For this review, take the finished solid that the model builds, in its own axes (mm). Face numbers are marked on the shaded views. Give positions to 0.01 mm unless a question says otherwise; leave off trailing zeros. Loops run counter-clockwise (first coordinate to the right, second up) from the corner with the lowest first, then second, coordinate; pieces in that order, holes last. Notation, with made-up numbers: (31, 45) - (40, 45) arc R35 cw to (40, 82) - close; hole circle Ø8 at (2.5, -32.75). An arc over 180 degrees is marked (long way). Put each result on its own line as item: value. Start each with the question number.
from build123d import *

# Parameters (mm, degrees)
SKETCH1_W             = 9.525
SKETCH1_H             = 142.875
BOSS_EXTRUDE1_DEPTH   = 1.5875
BOSS_EXTRUDE1_2_DEPTH = 1.5875
SKETCH2_W             = 4.7625
SKETCH2_H             = 142.875
BOSS_EXTRUDE2_DEPTH   = 59.055
SKETCH3_W             = 127
SKETCH3_H             = 38.1
CUT_EXTRUDE1_DEPTH    = 164.834934713
SKETCH4_R             = 26.2255
SKETCH4_R_2           = 22.225
BOSS_EXTRUDE3_DEPTH   = 4.7625
FILLET1_R             = 6.35
FILLET4_R             = 6.35
SKETCH5_W             = 44.45
SKETCH5_H             = 1.5875
BOSS_EXTRUDE4_DEPTH   = 142.875


with BuildPart() as part:
    # Sketch1 → Boss-Extrude1 (new body)
    with BuildSketch(Plane(origin=(0, 0, 0), x_dir=(1, 0, 0), z_dir=(0, 1, 0))):
        with Locations((4.7625, 71.4375)):
            Rectangle(SKETCH1_W, SKETCH1_H)
    extrude(amount=BOSS_EXTRUDE1_DEPTH)



with BuildPart() as body_2:
    # Sketch1 → Boss-Extrude1 2 (new body)
    with BuildSketch(Plane(origin=(0, 0, 0), x_dir=(1, 0, 0), z_dir=(0, 1, 0))):
        with Locations((47.6885, 71.4375)):
            Rectangle(SKETCH1_W, SKETCH1_H)
    extrude(amount=BOSS_EXTRUDE1_2_DEPTH)


with BuildPart() as part_1:
    add(part.part)

    add(body_2.part)  # Boss-Extrude2 merges body 2
    # Sketch2 → Boss-Extrude2 (add)
    with BuildSketch(Plane(origin=(0, 1.5875, 0), x_dir=(1, 0, 0), z_dir=(0, 1, 0))):
        with Locations((2.38125, 71.4375)):
            Rectangle(SKETCH2_W, SKETCH2_H)
        with Locations((50.06975, 71.4375)):
            Rectangle(SKETCH2_W, SKETCH2_H)
    extrude(amount=BOSS_EXTRUDE2_DEPTH)

    # Sketch3 → Cut-Extrude1 (cut, through all)
    with BuildSketch(Plane.ZY):
        with Locations((-71.4375, 30.32125)):
            Rectangle(SKETCH3_W, SKETCH3_H)
    extrude(amount=-CUT_EXTRUDE1_DEPTH, mode=Mode.SUBTRACT)

    # Sketch4 → Boss-Extrude3 (add)
    with BuildSketch(Plane(origin=(0, 0, -142.875), x_dir=(-1, 0, 0), z_dir=(0, 0, -1))):
        with Locations((-26.2255, 30.32125)):
            Circle(SKETCH4_R)
        with Locations((-26.2255, 30.32125)):
            Circle(SKETCH4_R_2, mode=Mode.SUBTRACT)
    extrude(amount=-BOSS_EXTRUDE3_DEPTH)

    # Fillet1
    # the kernel refuses this fillet: 6.35 mm, written as the material it takes off along each edge
    with BuildSketch(Plane(origin=(52.451, 0, -158.75), x_dir=(0, 1, 0), z_dir=(0, 0, 1)), Plane(origin=(0, 0, -158.75), x_dir=(1, 0, 0), z_dir=(0, 0, 1))) as fillet1_piece_1:
        with BuildLine():
            CenterArc((FILLET1_R, FILLET1_R), FILLET1_R, 180, 90)
            Line((0, FILLET1_R), (-FILLET1_R * 0.02, FILLET1_R))
            Line((-FILLET1_R * 0.02, FILLET1_R), (-FILLET1_R * 0.02, -FILLET1_R * 0.02))
            Line((-FILLET1_R * 0.02, -FILLET1_R * 0.02), (FILLET1_R, -FILLET1_R * 0.02))
            Line((FILLET1_R, -FILLET1_R * 0.02), (FILLET1_R, 0))
        make_face()
    extrude(amount=174.625, mode=Mode.SUBTRACT)
    with BuildSketch(Plane(origin=(0, 60.6425, -158.245902655), x_dir=(1, 0, 0), z_dir=(0, 0, 1))) as fillet1_piece_2:
        with BuildLine():
            CenterArc((6.35, -6.148361062), FILLET1_R, 104.477512186, 75.522487814)
            Line((0, -6.148361062), (-0.127, -6.148361062))
            Line((-0.127, -6.148361062), (-0.127, 0))
            Line((-0.127, 0), (0, 0.127))
            ThreePointArc((0, 0.127), (2.38125, 0.127), (4.73075, 0.122967221))
            Line((4.73075, 0.122967221), (4.7625, 0))
        make_face()
    extrude(amount=173.616805311, mode=Mode.SUBTRACT)
    with BuildSketch(Plane(origin=(52.451, 60.6425, -158.245902655), x_dir=(0, -1, 0), z_dir=(0, 0, 1))) as fillet1_piece_3:
        with BuildLine():
            CenterArc((6.148361062, -6.35), FILLET1_R, 90, 75.522487814)
            Line((0, -4.7625), (-0.122967221, -4.73075))
            ThreePointArc((-0.122967221, -4.73075), (-0.127, -2.38125), (-0.127, 0))
            Line((-0.127, 0), (0, 0.127))
            Line((0, 0.127), (6.148361062, 0.127))
            Line((6.148361062, 0.127), (6.148361062, 0))
        make_face()
    extrude(amount=173.616805311, mode=Mode.SUBTRACT)

    # Fillet4
    fillet4_edges = [part_1.edges().sort_by_distance(p)[0] for p in [
        (2.38125, 11.27125, -134.9375),
        (2.38125, 49.37125, -134.9375),
        (2.38125, 49.37125, -7.9375),
        (2.38125, 11.27125, -7.9375),
        (50.06975, 49.37125, -134.9375),
        (50.06975, 49.37125, -7.9375),
        (50.06975, 11.27125, -7.9375),
        (50.06975, 11.27125, -134.9375),
    ]]
    fillet(fillet4_edges, radius=FILLET4_R)

    # Sketch5 → Boss-Extrude4 (add)
    with BuildSketch(Plane.XY):
        with Locations((26.2255, 58.26125)):
            Rectangle(SKETCH5_W, SKETCH5_H)
    extrude(amount=-BOSS_EXTRUDE4_DEPTH)


solid = part_1.part
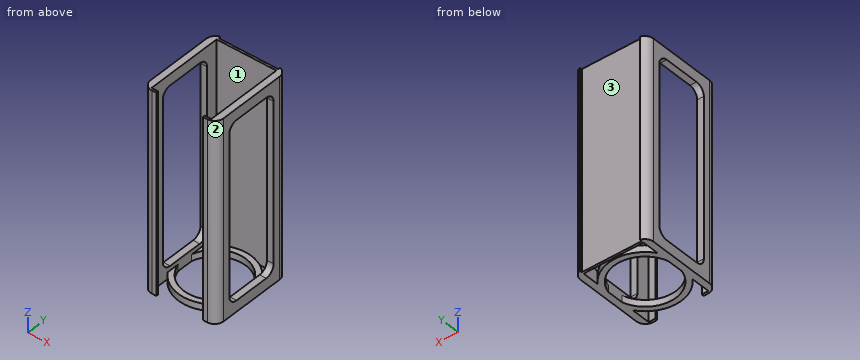
1) Take a section at D-D on y = 47. State the section outline as (x, z) points (1 decimal).
2) Wall thickness on probe 1 along X at (y, z) = (49.5, -40); probe 2 along Y at (x, z) = (6.5, -71.5) (1 decimal); probe 3 along Y at (x, z) = (14, -12) (1 decimal): over which ranges is each line inside the solid? List them lowest first.
3) Take a section at C-C on x = 19. State the section outline as (y, z) points (1 decimal).
4) Take a section at B-B on y = 33. State the section outline as (x, z) points (1 decimal), and give its area (3 significant figures).
5) Take a section at A-A on z = -75. State how many separate pieces and enclosed holes the cut face has, and give its area (3 significant figures).
6) Mouldability with a two-part tool opening along Y and no side actions: class the marked faces 1, 2 and 3 as released by +Y, released by -Y, zero draft, split by the parting line, or undercut.
7) Insertion check: P1, Ø2.5, axis at x = 3.5, z = -55.5, coming from the +Y side; P2, Ø10, axis at y = 49.5, z = -93, coming from the -X side; P3, Ø10, axis at x = 33, y = 10.5, coming from the +Z side; P4, Ø1.4, axis at x = 44.5, z = -86.5, coming from the +Y side (3 decimals). Each pin has a flat end and moves straight along its axis. Give the tip position at first contact, or say it passes through.
Answers follow:
1. outline: (0, -142.9) - (4.8, -142.9) - (4.8, -133.5) - (0, -133.5) - close; (0, -9.3) - (4.8, -9.3) - (4.8, 0) - (0, 0) - close; (6, -142.9) - (11.5, -142.9) - (11.5, -138.1) - (6, -138.1) - close; (40.9, -142.9) - (46.5, -142.9) - (46.5, -138.1) - (40.9, -138.1) - close; (47.7, -142.9) - (52.5, -142.9) - (52.5, -133.5) - (47.7, -133.5) - close; (47.7, -9.3) - (52.5, -9.3) - (52.5, 0) - (47.7, 0) - close
2. probe 1: 0 to 4.76, 47.69 to 52.45
2. probe 2: 0 to 1.6, 57.5 to 59.1
2. probe 3: 57.5 to 59.1
3. outline: (5.1, -142.9) - (9.3, -142.9) - (9.3, -138.1) - (5.1, -138.1) - close; (51.3, -142.9) - (55.5, -142.9) - (55.5, -138.1) - (51.3, -138.1) - close; (57.5, -142.9) - (59.1, -142.9) - (59.1, 0) - (57.5, 0) - close
4. outline: (0, -142.9) - (4.8, -142.9) - (4.8, -134.9) - (0, -134.9) - close; (0, -7.9) - (4.8, -7.9) - (4.8, 0) - (0, 0) - close; (47.7, -142.9) - (52.5, -142.9) - (52.5, -134.9) - (47.7, -134.9) - close; (47.7, -7.9) - (52.5, -7.9) - (52.5, 0) - (47.7, 0) - close
4. area: 151 mm2
5. separate pieces: 3
5. enclosed holes: 0
5. area: 266 mm2
6. face 1: undercut
6. face 2: released by -Y
6. face 3: released by +Y
7. P1: y = 60.64
7. P2: x = 0
7. P3: z = -138.11
7. P4: y = 59.055
